```python
from build123d import *

# Parameters (mm, degrees)
SKETCH_1_W          = 60
SKETCH_1_H          = 40
EXTRUDE_1_DEPTH     = 40
SKETCH_2_W          = 40
SKETCH_2_H          = 36
CUT_EXTRUDE_1_DEPTH = 57
CUT_EXTRUDE_2_REACH = 84.462
SKETCH_3_R          = 1.5
SKETCH_4_R          = 0.75
CUT_EXTRUDE_3_DEPTH = 38
SKETCH_5_R          = 12
CUT_EXTRUDE_4_DEPTH = 83.462112512


with BuildPart() as part:
    # 草图1 → 凸台-拉伸1 (new body)
    with BuildSketch(Plane.XY):
        with Locations((30, 20)):
            Rectangle(SKETCH_1_W, SKETCH_1_H)
    extrude(amount=EXTRUDE_1_DEPTH)

    # 草图2 → 切除-拉伸1 (cut)
    with BuildSketch(Plane.ZY):
        with Locations((20, 20)):
            Rectangle(SKETCH_2_W, SKETCH_2_H)
    extrude(amount=-CUT_EXTRUDE_1_DEPTH, mode=Mode.SUBTRACT)

    # 草图3 → 切除-拉伸2 (cut, up to next)
    with BuildSketch(Plane(origin=(60, 0, 0), x_dir=(0, 0, -1), z_dir=(1, 0, 0)), mode=Mode.PRIVATE) as cut_extrude_2_sk1:
        with Locations((-20, 20)):
            Circle(SKETCH_3_R)
    cut_extrude_2_tool1 = extrude(cut_extrude_2_sk1.sketch, amount=-CUT_EXTRUDE_2_REACH, mode=Mode.PRIVATE) & part.part
    add(cut_extrude_2_tool1.solids().sort_by_distance((60, 20, 20))[0], mode=Mode.SUBTRACT)

    # 草图4 → 切除-拉伸3 (cut)
    with BuildSketch(Plane(origin=(60, 0, 0), x_dir=(0, 0, -1), z_dir=(1, 0, 0))):
        with Locations((-20, 27)):
            Circle(SKETCH_4_R)
        with Locations((-13, 20)):
            Circle(SKETCH_4_R)
        with Locations((-20, 13)):
            Circle(SKETCH_4_R)
        with Locations((-27, 20)):
            Circle(SKETCH_4_R)
    extrude(amount=-CUT_EXTRUDE_3_DEPTH, mode=Mode.SUBTRACT)

    # 草图5 → 切除-拉伸4 (cut, through all)
    with BuildSketch(Plane(origin=(0, 40, 0), x_dir=(1, 0, 0), z_dir=(0, 1, 0))):
        with Locations(Location((20, -20, 0), (0, 0, 270))):
            Circle(SKETCH_5_R)
    extrude(amount=-CUT_EXTRUDE_4_DEPTH, mode=Mode.SUBTRACT)


solid = part.part
```
Read the model definition and answer for the solid it produces. Units are mm, in the model's axes. A direction names the side the tool comes from. Coordinates: 2 decimals unless noted, no trailing zeros. Write each loop counter-clockwise with the first axis right and the second up, starting at its lowest first coordinate (ties: lowest second). Pieces come first, ordered by that corner, then holes. Notation, with made-up numbers: (77, 10) -> (115, 10) arc R20 ccw to (115, 39) -> close; hole circle Ø8 at (-6, 54). An arc over 180 degrees is marked (long way). Write item = value, one per line.
(1) Section C-C on z = 20 is taken. Write down the section's boundary in (x, y), plus the area to 3 significant figures.
From the geometry:
outline = (0, 0) -> (8, 0) -> (8, 2) -> (0, 2) -> close; (0, 38) -> (8, 38) -> (8, 40) -> (0, 40) -> close; (32, 0) -> (60, 0) -> (60, 12.25) -> (57, 12.25) -> (57, 2) -> (32, 2) -> close; (32, 38) -> (57, 38) -> (57, 27.75) -> (60, 27.75) -> (60, 40) -> (32, 40) -> close; (57, 13.75) -> (60, 13.75) -> (60, 18.5) -> (57, 18.5) -> close; (57, 21.5) -> (60, 21.5) -> (60, 26.25) -> (57, 26.25) -> close
area = 234 mm2
(2) Section D-D on x = 20 is taken. Write down the section's boundary in (y, z).
From the geometry:
outline = (0, 0) -> (2, 0) -> (2, 8) -> (0, 8) -> close; (0, 32) -> (2, 32) -> (2, 40) -> (0, 40) -> close; (38, 0) -> (40, 0) -> (40, 8) -> (38, 8) -> close; (38, 32) -> (40, 32) -> (40, 40) -> (38, 40) -> close
(3) For a pull along Y with two mould halves and no side action, classify faces 1 (the face through (60, 24, 20)), 2 (the face through (36, 0, 20)), 3 (the face through (34, 2, 20)), 4 (the face through (34, 38, 20)) as +Y half, -Y half, draft (parallel to the pull), parting line (faces both ways), or undercut.
From the geometry:
face_1 = draft
face_2 = -Y half
face_3 = undercut
face_4 = undercut
(4) Given pin 1 Ø1.8 at (y, z) = (20, 20) entering from -X; pin 2 Ø20 at (x, z) = (20, 28.5) entering from -Y; pin 3 Ø1.7 at (y, z) = (20, 13) entering from -X, each flat-ended and moving along its own axis, determine where each tip first touches the part or whether it passes through.
From the geometry:
pin_1 = through
pin_2 = 0
pin_3 = 57
(5) Straight lines are drawn through the part: L1, parallel to Y at x = 57.8, z = 20; L2, parallel to Y at x = 12, z = 36.5; L3, parallel to Y at x = 58, z = 27. For each, find the intervals that lie inside material, in ascending order. Write a range as from..to.
From the geometry:
L1 = 0..12.25, 13.75..18.5, 21.5..26.25, 27.75..40
L2 = 0..2, 38..40
L3 = 0..19.25, 20.75..40
(6) Which of the six approach directions +Z, -Z, +X, -X, +Y, -Y give full straight-line access (tool end or side, diameter ignored) to faces 5 (the face through (0, 39, 20)), 6 (the face through (57, 16, 20))?
From the geometry:
face_5 = +Z, -Z, -X, +Y, -Y
face_6 = +Z, -Z, -X
(7) Section B-B on x = 34 is taken. Write down the section's boundary in (y, z).
From the geometry:
outline = (0, 0) -> (2, 0) -> (2, 40) -> (0, 40) -> close; (38, 0) -> (40, 0) -> (40, 40) -> (38, 40) -> close
(8) Section A-A on y = 27 is taken. Write down the section's boundary in (x, z), plus the area to 4 significant figures.
From the geometry:
outline = (57, 0) -> (60, 0) -> (60, 19.25) -> (57, 19.25) -> close; (57, 20.75) -> (60, 20.75) -> (60, 40) -> (57, 40) -> close
area = 115.5 mm2
